For this review, use the dimensioned drawing (mm, ordinates from the lowest corner) and the shaded views. A direction names the side the tool comes from. Coordinates: 2 decimals unless noted, no trailing zeros. Write each loop counter-clockwise with the first axis right and the second up, starting at its lowest first coordinate (ties: lowest second). Pieces come first, ordered by that corner, then holes.
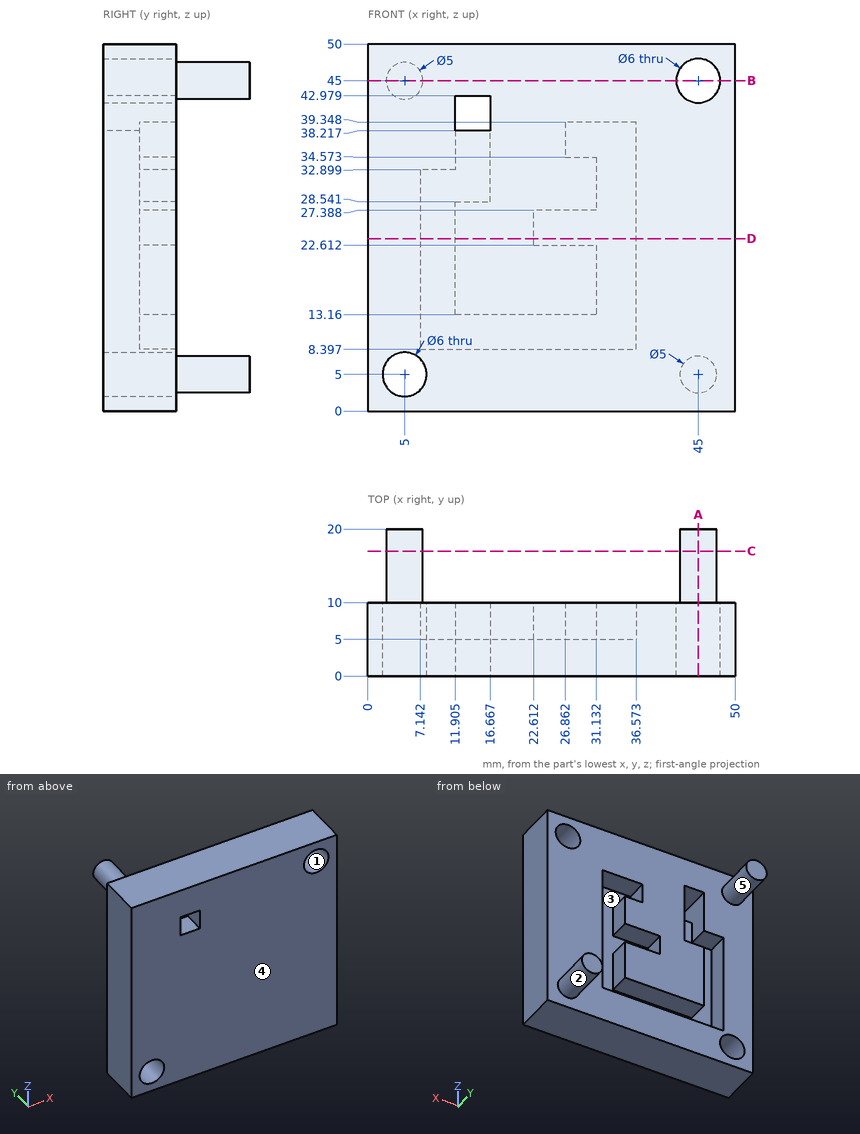
Item 1: Machinability: for the marked faces 1 and 2, which of the approach directions +Z, -Z, +X, -X, +Y, -Y give a long, thin tool a straight path to every point of the face, cutting with its end or side? Answer none if there is none.
Solved:
face 1: +Y, -Y
face 2: +Y
Item 2: Take a section at C-C, the plane y = 17. Write out the cut boundary in (x, z).
Solved:
outline: circle Ø5 at (5, 45); circle Ø5 at (45, 5)
Item 3: Take a section at D-D, the plane z = 23.5. Write out the cut boundary in (x, y) (1 decimal).
Solved:
outline: (0, 0) - (50, 0) - (50, 10) - (36.6, 10) - (36.6, 5) - (22.6, 5) - (22.6, 10) - (11.9, 10) - (11.9, 5) - (7.1, 5) - (7.1, 10) - (0, 10) - close
Item 4: For pin 1 (5.5 mm diameter, centred on x = 5, z = 5, fed in from +Y); pin 2 (1 mm diameter, centred on x = 32.5, z = 34, fed in from +Y); pin 3 (15 mm diameter, centred on x = 27.5, z = 26, fed in from +Y); pin 4 (6 mm diameter, centred on y = 16, z = 9.5, fed in from +X), all flat-tipped, find the tip position at first contact; note any pin that passes through.
Solved:
pin 1: passes through
pin 2: stops at y = 5
pin 3: stops at y = 10
pin 4: stops at x = 47
Item 5: Take a section at A-A, the plane x = 45. Write out the cut boundary in (y, z), plus the area to 3 significant figures.
Solved:
outline: (0, 0) - (10, 0) - (10, 2.5) - (20, 2.5) - (20, 7.5) - (10, 7.5) - (10, 42) - (0, 42) - close; (0, 48) - (10, 48) - (10, 50) - (0, 50) - close
area: 490 mm2
Item 6: To check wall thickness, follow line 1 along X through (y, z) = (7, 27) (1 decimal); line 2 along Z through (x, y) = (45, 6.5); line 3 along X through (y, z) = (6.25, 31). State the ranges of each line that lie inside material, in increasing order.
Solved:
line 1: x = 0 to 7.1, 11.9 to 22.6, 36.6 to 50
line 2: z = 0 to 42, 48 to 50
line 3: x = 0 to 7.14, 16.67 to 31.13, 36.57 to 50
Item 7: Take a section at B-B, the plane z = 45. Write out the cut boundary in (x, y), plus the area to 3 significant figures.
Solved:
outline: (0, 0) - (42, 0) - (42, 10) - (7.5, 10) - (7.5, 20) - (2.5, 20) - (2.5, 10) - (0, 10) - close; (48, 0) - (50, 0) - (50, 10) - (48, 10) - close
area: 490 mm2
Item 8: Mouldability with a two-part tool opening along X and no side actions: class the marked faces 3, 4 and 5 as pulls with the +X half, pulls with the -X half, needs draft (parallel to the pull), parting line crosses it, or undercut.
Solved:
face 3: undercut
face 4: needs draft
face 5: parting line crosses it
